```python
from build123d import *

# Parameters (mm, degrees)
SKETCH1_R                            = 9
SKETCH1_R_2                          = 7
EXTRUDE_THIN1_DEPTH                  = 380
BOSS_EXTRUDE1_REACH                  = 382.213
BOSS_EXTRUDE1_END_RADIUS             = 7
SKETCH2_R                            = 1.5
BOSS_EXTRUDE1_DIRECTION_2_REACH      = 382.213
BOSS_EXTRUDE1_DIRECTION_2_END_RADIUS = 7
BOSS_EXTRUDE2_START                  = 8
SKETCH3_R                            = 1.5
BOSS_EXTRUDE2_DEPTH                  = 8


with BuildPart() as part:
    # Sketch1 → Extrude-Thin1 (new body)
    with BuildSketch(Plane(origin=(0, 0, 0), x_dir=(1, 0, 0), z_dir=(0, 1, 0))):
        Circle(SKETCH1_R)
        Circle(SKETCH1_R_2, mode=Mode.SUBTRACT)
    extrude(amount=EXTRUDE_THIN1_DEPTH)

    # Boss-Extrude1: up to this cylinder (the profile starts inside it)
    boss_extrude1_end = Plane(origin=(0, 4.5, 0), z_dir=(0, -1, 0)) * Cylinder(BOSS_EXTRUDE1_END_RADIUS, 779.426, mode=Mode.PRIVATE)
    # Sketch2 → Boss-Extrude1 (add, up to the surface)
    with BuildSketch(Plane(origin=(0, 0, 0), x_dir=(0, 0, -1), z_dir=(1, 0, 0)), mode=Mode.PRIVATE) as boss_extrude1_sk1:
        with Locations((0, 4.5)):
            Circle(SKETCH2_R)
    boss_extrude1_tool1 = extrude(boss_extrude1_sk1.sketch, amount=BOSS_EXTRUDE1_REACH, mode=Mode.PRIVATE) & boss_extrude1_end
    add(boss_extrude1_tool1.solids().sort_by_distance((0, 4.5, 0))[0])

    # Boss-Extrude1 direction 2: up to this cylinder (the profile starts inside it)
    boss_extrude1_direction_2_end = Plane(origin=(0, 4.5, 0), z_dir=(0, -1, 0)) * Cylinder(BOSS_EXTRUDE1_DIRECTION_2_END_RADIUS, 779.426, mode=Mode.PRIVATE)
    # Sketch2 → Boss-Extrude1 direction 2 (add, up to the surface)
    with BuildSketch(Plane(origin=(0, 0, 0), x_dir=(0, 0, -1), z_dir=(1, 0, 0)), mode=Mode.PRIVATE) as boss_extrude1_direction_2_sk1:
        with Locations((0, 4.5)):
            Circle(SKETCH2_R)
    boss_extrude1_direction_2_tool1 = extrude(boss_extrude1_direction_2_sk1.sketch, amount=-BOSS_EXTRUDE1_DIRECTION_2_REACH, mode=Mode.PRIVATE) & boss_extrude1_direction_2_end
    add(boss_extrude1_direction_2_tool1.solids().sort_by_distance((0, 4.5, 0))[0])

    # Sketch3 → Boss-Extrude2 (add)
    with BuildSketch(Plane(origin=(0, 0, 0), x_dir=(0, 0, -1), z_dir=(1, 0, 0)).offset(BOSS_EXTRUDE2_START)):
        with Locations(Location((0, 30, 0), (0, 0, 180))):
            Circle(SKETCH3_R)
    extrude(amount=BOSS_EXTRUDE2_DEPTH)


solid = part.part
```
Model file for the job. Use its own axes, mm. Coordinates: 2 decimals unless noted, no trailing zeros. Order: outer loops, then holes, each group sorted by start corner. A loop starts at its lowest first (then second) coordinate and runs counter-clockwise, first axis right, second up. Notation, with made-up numbers: (48, -38.5) -> (77, -38.5) arc R22 ccw to (77, -17.5) -> close; hole circle Ø11 at (68, -33). An arc over 180 degrees is marked (long way). Answer as a JSON object with one key per item and string values. Group by question number.
1) Flat gauge pins, fed straight in: pin 1 (4 mm diameter, centred on x = -3, y = 300.5, fed in from -Z); pin 2 (4 mm diameter, centred on x = -2.5, y = 215, fed in from -Z); pin 3 (1.5 mm diameter, centred on x = -5.5, y = 81.5, fed in from +Z). Where does each tip first touch, or does it go through?
2) Cut at A-A, the plane x = 0. Write the cut outline in (y, z), then the cut area to 3 significant figures.
3) Pull direction Z, two halves, no side cores. Call faces 1 (the face through (0, 380, 7.3)), 2 (the face through (6.677, 187.34, -2.103)), 3 (the face through (-1.172, 187.34, -8.923)): +Z half, -Z half, draft (parallel to the pull), parting line (faces both ways), or undercut.
4) Drill centre lines: L1, parallel to X at y = 144.5, z = 0; L2, parallel to Z at x = -3, y = 328. Where is each one in solid material? Low to high.
5) Cut at B-B, the plane y = 83.5. Write the cut outline in (x, z), then the cut area to 3 significant figures.
Check values:
{
 "1": {"pin 1": "stops at z = -8.94", "pin 2": "stops at z = -8.99", "pin 3": "stops at z = 7.64"},
 "2": {"outline": "(0, -9) -> (380, -9) -> (380, -7) -> (0, -7) -> close; (0, 7) -> (380, 7) -> (380, 9) -> (0, 9) -> close; circle Ø3 at (4.5, 0)", "area": "1,530 mm²"},
 "3": {"face 1": "draft", "face 2": "undercut", "face 3": "parting line"},
 "4": {"L1": "x = -9 to -7, 7 to 9", "L2": "z = -8.49 to -6.32, 6.32 to 8.49"},
 "5": {"outline": "circle Ø18 at (0, 0); hole circle Ø14 at (0, 0)", "area": "101 mm²"}
}
